from build123d import *

# Parameters (mm, degrees)
CUT_EXTRUDE1_REACH = 16.523
SKETCH2_W          = 4.904374576
SKETCH2_H          = 1.390216618
SKETCH2_W_2        = 1.390216618
SKETCH2_H_2        = 4.904374576


with BuildPart() as part:
    # Sketch1 → Revolve1 (revolve)
    with BuildSketch(Plane.XY, mode=Mode.PRIVATE) as revolve1_sk:
        with BuildLine():
            Line((0, 0), (0, 12.7))
            Line((0, 12.7), (0, 13.8684))
            Line((0, 13.8684), (0, 16.128443135))
            add(Edge.make_bspline(
                [(0, 16.128443135), (2.158115005, 15.748885895), (3.048, 13.8684)],
                knots=[0, 0, 0, 1, 1, 1], degree=2))
            Line((3.048, 13.8684), (3.048, 12.7))
            Line((3.048, 12.7), (1.5, 12.7))
            Line((1.5, 12.7), (1.5, 0))
            Line((1.5, 0), (0, 0))
        make_face()
    revolve(revolve1_sk.sketch.rotate(Axis((0, 18.881175956, 0), (0, -1, 0)), 90), axis=Axis((0, 18.881175956, 0), (0, -1, 0)))

    # Sketch2 → Cut-Extrude1 (cut, up to next)
    with BuildSketch(Plane(origin=(0, 13.8684, 0), x_dir=(-1, 0, 0), z_dir=(0, -1, 0)), mode=Mode.PRIVATE) as cut_extrude1_sk1:
        Rectangle(SKETCH2_W, SKETCH2_H)
    cut_extrude1_tool1 = extrude(cut_extrude1_sk1.sketch, amount=-CUT_EXTRUDE1_REACH, mode=Mode.PRIVATE) & part.part
    # Sketch2 → Cut-Extrude1 (cut, up to next)
    with BuildSketch(Plane(origin=(0, 13.8684, 0), x_dir=(-1, 0, 0), z_dir=(0, -1, 0)), mode=Mode.PRIVATE) as cut_extrude1_sk2:
        Rectangle(SKETCH2_W_2, SKETCH2_H_2)
    cut_extrude1_tool2 = extrude(cut_extrude1_sk2.sketch, amount=-CUT_EXTRUDE1_REACH, mode=Mode.PRIVATE) & part.part
    add(cut_extrude1_tool1.solids().sort_by_distance((0, 13.8684, 0))[0], mode=Mode.SUBTRACT)
    add(cut_extrude1_tool2.solids().sort_by_distance((0, 13.8684, 0))[0], mode=Mode.SUBTRACT)


solid = part.part
The listing builds one solid part. Answer for the finished solid, in the listing's coordinates (mm). A direction names the side the tool comes from. Give positions to 0.01 mm unless a question says otherwise; leave off trailing zeros. Order: outer loops, then holes, each group sorted by start corner. A loop starts at its lowest first (then second) coordinate and runs counter-clockwise, first axis right, second up. Notation, with made-up numbers: (-34, -1) - (8, -1) arc R23 cw to (8, 16) - close; hole circle Ø1 at (-18, 78.5). An arc over 180 degrees is marked (long way). One line per item, written item: value. Start each with the question number.
1) Find the intervals of material crossed by L1, parallel to Z at x = -1.25, y = 14.75; L2, parallel to X at y = 15, z = 0.75; L3, parallel to X at y = 14.5, z = -0.25, in increasing order.
2) The mould has two halves that part along Z. Classify faces 4 (the face through (-0.45, 6.26, 1.43)), 5 (the face through (1, 15, -0.695)), 6 (the face through (0, 0, 0)), 7 (the face through (-0.695, 15, 1)): released by +Z, released by -Z, zero draft, split by the parting line, or undercut.
3) A tool of negligible diameter and unlimited length cuts with its end or side. For faces 1 (the face through (-3.02, 13.28, -0.4)), 2 (the face through (1.3, 12.7, 1.3)), 3 (the face through (2.452, 14.3, 0)), from which of +Z, -Z, +X, -X, +Y, -Y can it reach the whole face along a straight path? Write none if from no direction.
4) Given pin 1 Ø1.9 at (y, z) = (14.5, -1.5) entering from -X; pin 2 Ø1.5 at (y, z) = (9.5, 2.5) entering from -X; pin 3 Ø1.4 at (y, z) = (15, 1.5) entering from -X; pin 4 Ø1.4 at (y, z) = (15, -1.5) entering from +X, each flat-ended and moving along its own axis, determine where each tip first touches the part or whether it passes through.
5) A cutting plane is placed at A-A on y = 13. Give the vertices of the cut face in (x, z).
6) A cutting plane is placed at B-B on y = 5.5. Give the vertices of the cut face in (x, z).
Answer sheet:
1. L1: z = -2.16 to -0.7, 0.7 to 2.16
1. L2: x = -2.14 to -0.7, 0.7 to 2.14
1. L3: x = -2.67 to -2.45, 2.45 to 2.67
2. face 4: split by the parting line
2. face 5: undercut
2. face 6: zero draft
2. face 7: undercut
3. face 1: +Y, -Y
3. face 2: -Y
3. face 3: +Y
4. pin 1: stops at x = -2.94
4. pin 2: passes through
4. pin 3: stops at x = -2.5
4. pin 4: stops at x = 2.5
5. outline: circle Ø6.1 at (0, 0)
6. outline: circle Ø3 at (0, 0)
